Source: CAD feature listing. Evaluate the final solid. Frame: model axes, mm. Face numbers are marked on the shaded views. Give positions to 0.01 mm unless a question says otherwise; leave off trailing zeros. Order: outer loops, then holes, each group sorted by start corner. A loop starts at its lowest first (then second) coordinate and runs counter-clockwise, first axis right, second up.
```python
from build123d import *

# Parameters (mm, degrees)
P_IDAT_VYSUNUT_M1_DEPTH  = 5.6
SKO_EPINA1_T             = 1.8
P_IDAT_VYSUNUT_M3_DEPTH  = 5.15
P_IDAT_VYSUNUT_M4_DEPTH  = 7.4
P_IDAT_VYSUNUT_M5_DEPTH  = 1.5
SKICA14_W                = 49.9
SKICA14_H                = 0.995009232
P_IDAT_VYSUNUT_M6_DEPTH  = 1.5
SKICA15_R                = 5.4
SKICA15_W                = 3
SKICA15_H                = 9
P_IDAT_VYSUNUT_M7_DEPTH  = 5.6
SKICA16_R                = 2
ODEBRAT_VYSUNUT_M1_DEPTH = 5.75
ZKOSEN_1_SIZE            = 1
SKICA17_W                = 24
SKICA17_H                = 13.4
ODEBRAT_VYSUNUT_M2_DEPTH = 1.6
ODEBRAT_VYSUNUT_M3_REACH = 442.031
SKICA23_R                = 2
ODEBRAT_VYSUNUT_M4_DEPTH = 5.7
SKICA24_R                = 2
ODEBRAT_VYSUNUT_M5_DEPTH = 5.7
SKICA25_R                = 6.25
ODEBRAT_VYSUNUT_M6_DEPTH = 1.5


with BuildPart() as part:
    # Skica3 → P_idat vysunut_m1 (new body)
    with BuildSketch(Plane.XY):
        Polygon((2.412545276, -4), (412.692715215, -4), (412.692715215, -118.191389918), (412.654731358, -118.229366948), (404.717731358, -118.229366948), (402.336688893, -120.609981536), (12.768122748, -120.609981536), (10.387229089, -118.22921813), (2.450229089, -118.22921813), (2.412545276, -118.191536378), align=None)
    extrude(amount=P_IDAT_VYSUNUT_M1_DEPTH)

    # Sko_epina1
    sko_epina1_openings = [part.faces().sort_by_distance(p)[0] for p in [
        (207.552632266, -62.25279763, 5.6),
    ]]
    offset(amount=SKO_EPINA1_T, openings=sko_epina1_openings, kind=Kind.INTERSECTION)



with BuildPart() as body_2:
    # Skica7 → P_idat vysunut_m3 (new body)
    with BuildSketch(Plane.XY.offset(5.6)):
        Polygon((-6.587454724, 5), (-6.587454724, -121.919602656), (-1.277548758, -127.22921813), (6.659451242, -127.22921813), (9.040344901, -129.609981536), (406.06413722, -129.609981536), (408.445179685, -127.229366948), (416.382179685, -127.229366948), (421.692715215, -121.919785731), (421.692715215, 5), align=None)
        Polygon((-3.787454724, 2.2), (-3.787454724, -120.759759814), (-0.11779565, -124.42921813), (7.81920435, -124.42921813), (10.200098009, -126.809981536), (404.904486629, -126.809981536), (407.285529094, -124.429366948), (415.222529094, -124.429366948), (418.892715215, -120.759840367), (418.892715215, 2.2), align=None, mode=Mode.SUBTRACT)
    extrude(amount=P_IDAT_VYSUNUT_M3_DEPTH)


with BuildPart() as part_1:
    add(part.part)

    add(body_2.part)  # P_idat vysunut_m4 merges body 2
    # Skica8 → P_idat vysunut_m4 (add)
    with BuildSketch(Plane(origin=(0, 0, 5.6), x_dir=(-1, 0, 0), z_dir=(0, 0, -1))):
        Polygon((-421.692715215, 5), (6.587454724, 5), (6.587454724, -121.919602656), (1.277548758, -127.22921813), (-6.659451242, -127.22921813), (-9.040344901, -129.609981536), (-406.06413722, -129.609981536), (-408.445179685, -127.229366948), (-416.382179685, -127.229366948), (-421.692715215, -121.919785731), align=None)
        Polygon((-0.612545276, -2.2), (-0.612545276, -118.937149634), (-1.70467352, -120.02921813), (-9.64167352, -120.02921813), (-12.022567179, -122.409981536), (-403.082178558, -122.409981536), (-405.463221024, -120.029366948), (-413.400221024, -120.029366948), (-414.492715215, -118.93706908), (-414.492715215, -2.2), align=None, mode=Mode.SUBTRACT)
    extrude(amount=P_IDAT_VYSUNUT_M4_DEPTH)

    # Skica11 → P_idat vysunut_m5 (add)
    with BuildSketch(Plane.XY.offset(10.75)):
        Polygon((421.692715215, 5), (-6.587454724, 5), (-6.587454724, -121.919602656), (-1.277548758, -127.22921813), (6.659451242, -127.22921813), (9.040344901, -129.609981536), (406.06413722, -129.609981536), (408.445179685, -127.229366948), (416.382179685, -127.229366948), (421.692715215, -121.919785731), align=None)
        Polygon((420.052630246, 3.195009232), (-4.947369754, 3.195009232), (-4.947369754, -120.114611888), (-0.239981646, -124.821742467), (7.697018354, -124.821742467), (10.68042987, -127.804990768), (404.42405225, -127.804990768), (406.805094715, -125.424376181), (414.742094715, -125.424376181), (420.052630246, -120.114794964), align=None, mode=Mode.SUBTRACT)
    extrude(amount=P_IDAT_VYSUNUT_M5_DEPTH)

    # Skica14 → P_idat vysunut_m6 (add)
    with BuildSketch(Plane.XY.offset(10.75)):
        with Locations((157.582630246, 2.697504616)):
            Rectangle(SKICA14_W, SKICA14_H)
        with Locations((257.522630246, 2.697504616)):
            Rectangle(SKICA14_W, SKICA14_H)
        with Locations((257.52224106, -127.307486152)):
            Rectangle(SKICA14_W, SKICA14_H)
        with Locations((157.58224106, -127.307486152)):
            Rectangle(SKICA14_W, SKICA14_H)
    extrude(amount=P_IDAT_VYSUNUT_M6_DEPTH)

    # Skica15 → P_idat vysunut_m7 (add)
    with BuildSketch(Plane.XY):
        with Locations((3.968545276, -115.95421813)):
            Circle(SKICA15_R)
        with Locations((33.491545276, -69.050981536)):
            Circle(SKICA15_R)
        with Locations((411.197715215, -115.879366948)):
            Circle(SKICA15_R)
        with Locations((334.147715215, -53.972)):
            Circle(SKICA15_R)
        with Locations((36.401545276, 0)):
            Rectangle(SKICA15_W, SKICA15_H)
    extrude(amount=P_IDAT_VYSUNUT_M7_DEPTH)

    # Skica16 → Odebrat vysunut_m1 (cut)
    with BuildSketch(Plane.XY.offset(5.6)):
        with Locations((3.968545276, -115.95421813)):
            Circle(SKICA16_R)
        with Locations((33.491545276, -69.050981536)):
            Circle(SKICA16_R)
        with Locations((334.147715215, -53.972)):
            Circle(SKICA16_R)
        with Locations((411.197715215, -115.879366948)):
            Circle(SKICA16_R)
    extrude(amount=-ODEBRAT_VYSUNUT_M1_DEPTH, mode=Mode.SUBTRACT)

    # Zkosen_1
    zkosen_1_edges = [part_1.edges().sort_by_distance(p)[0] for p in [
        (8.049207709, -112.417525591, 0),
        (28.091545276, -69.050981536, 0),
        (407.069426922, -112.398384936, 0),
        (328.747715215, -53.972, 0),
    ]]
    chamfer(zkosen_1_edges, length=ZKOSEN_1_SIZE)

    # Skica17 → Odebrat vysunut_m2 (cut)
    with BuildSketch(Plane.XY.offset(5.6)):
        with Locations((36.401545276, -4.5)):
            Rectangle(SKICA17_W, SKICA17_H)
    extrude(amount=-ODEBRAT_VYSUNUT_M2_DEPTH, mode=Mode.SUBTRACT)

    # Odebrat vysunut_m3: up to this face of the body (flat: up to its plane)
    odebrat_vysunut_m3_end = Plane(part_1.part.faces().sort_by_distance((207.552630246, 5, 5.225))[0])
    # Skica18 → Odebrat vysunut_m3 (cut, up to the picked face)
    with BuildSketch(Plane.XZ.offset(4.5), mode=Mode.PRIVATE) as odebrat_vysunut_m3_sk1:
        with BuildLine():
            Line((33.651545276, 7.5), (39.151545276, 7.5))
            ThreePointArc((39.151545276, 7.5), (42.651545276, 4), (39.151545276, 0.5))
            Line((39.151545276, 0.5), (33.651545276, 0.5))
            ThreePointArc((33.651545276, 0.5), (30.151545276, 4), (33.651545276, 7.5))
        make_face()
    odebrat_vysunut_m3_tool1 = split(extrude(odebrat_vysunut_m3_sk1.sketch, amount=-ODEBRAT_VYSUNUT_M3_REACH, mode=Mode.PRIVATE), bisect_by=odebrat_vysunut_m3_end, keep=Keep.BOTH, mode=Mode.PRIVATE)
    add(odebrat_vysunut_m3_tool1.solids().sort_by(Axis((36.401545, -4.5, 4), (0, 1, 0)))[0], mode=Mode.SUBTRACT)

    # Skica23 → Odebrat vysunut_m4 (cut)
    with BuildSketch(Plane.ZY.offset(6.587454724)):
        with Locations((3.2, -18.459801328)):
            Circle(SKICA23_R)
        with Locations((3.2, -98.459801328)):
            Circle(SKICA23_R)
    extrude(amount=-ODEBRAT_VYSUNUT_M4_DEPTH, mode=Mode.SUBTRACT)

    # Skica24 → Odebrat vysunut_m5 (cut)
    with BuildSketch(Plane(origin=(421.692715215, 0, 0), x_dir=(0, 0, -1), z_dir=(1, 0, 0))):
        with Locations((-3.2, -18.459892866)):
            Circle(SKICA24_R)
        with Locations((-3.2, -98.459892866)):
            Circle(SKICA24_R)
    extrude(amount=-ODEBRAT_VYSUNUT_M5_DEPTH, mode=Mode.SUBTRACT)

    # Skica25 → Odebrat vysunut_m6 (cut)
    with BuildSketch(Plane(origin=(0, 0, -1.8), x_dir=(-1, 0, 0), z_dir=(0, 0, -1))):
        with Locations((-401.692715215, -15)):
            Circle(SKICA25_R)
        with Locations((-13.412545276, -15)):
            Circle(SKICA25_R)
        with Locations((-388.445179685, -109.609981536)):
            Circle(SKICA25_R)
        with Locations((-26.659451242, -109.609981536)):
            Circle(SKICA25_R)
    extrude(amount=-ODEBRAT_VYSUNUT_M6_DEPTH, mode=Mode.SUBTRACT)


solid = part_1.part
```
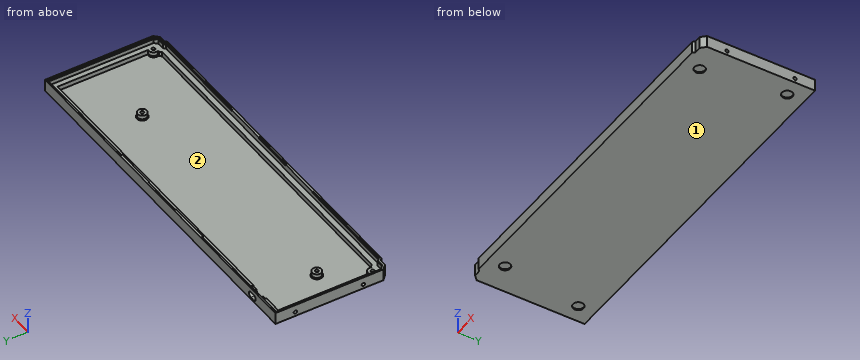
1) Material intervals for L1, parallel to Y at x = 213, z = 11 (3 decimals); L2, parallel to Y at x = 394.5, z = 0.5; L3, parallel to X at y = -105, z = 11.25, sorted ascending.
Report:
L1: y = -129.61 to -127.805, 3.195 to 5
L2: y = -129.61 to -120.61, -4 to 5
L3: x = -6.59 to -4.95, 420.05 to 421.69
2) Section query A-A, the plane x = 250.5. Return the cut outline in (y, z).
Report:
outline: (-129.61, -1.8) - (5, -1.8) - (5, 12.25) - (2.2, 12.25) - (2.2, 5.6) - (-4, 5.6) - (-4, 0) - (-120.61, 0) - (-120.61, 5.6) - (-126.81, 5.6) - (-126.81, 12.25) - (-129.61, 12.25) - close
3) Pin query (flat end, axial travel): pin 1 (1.2 mm diameter, centred on y = -19.5, z = 4, fed in from +X); pin 2 (20 mm diameter, centred on x = 388.45, y = -109.61, fed in from -Z); pin 3 (5.5 mm diameter, centred on x = 336.5, y = -54, fed in from +Z); pin 4 (2 mm diameter, centred on x = 164.5, y = -43.5, fed in from +Z). Return the tip coordinate at first contact, or that it passes through.
Report:
pin 1: stops at x = 415.99
pin 2: stops at z = -1.8
pin 3: stops at z = 5.6
pin 4: stops at z = 0
4) Draft query along X for the marked faces 1 and 2. Return one class per face: +X half, -X half, draft (parallel to the pull), parting line (faces both ways), or undercut.
Report:
face 1: draft
face 2: undercut
5) Section query C-C, the plane x = 56.5. Return the cut outline in (y, z) (3 decimals), and give its area (3 significant figures).
Report:
outline: (-129.61, -1.8) - (5, -1.8) - (5, 12.25) - (3.195, 12.25) - (3.195, 10.75) - (2.2, 10.75) - (2.2, 5.6) - (-4, 5.6) - (-4, 0) - (-120.61, 0) - (-120.61, 5.6) - (-126.81, 5.6) - (-126.81, 10.75) - (-127.805, 10.75) - (-127.805, 12.25) - (-129.61, 12.25) - close
area: 377 mm2
6) Section query B-B, the plane y = -34.5. Return the cut outline in (x, z).
Report:
outline: (-6.59, -1.8) - (421.69, -1.8) - (421.69, 12.25) - (420.05, 12.25) - (420.05, 10.75) - (418.89, 10.75) - (418.89, 5.6) - (412.69, 5.6) - (412.69, 0) - (2.41, 0) - (2.41, 5.6) - (-3.79, 5.6) - (-3.79, 10.75) - (-4.95, 10.75) - (-4.95, 12.25) - (-6.59, 12.25) - close
